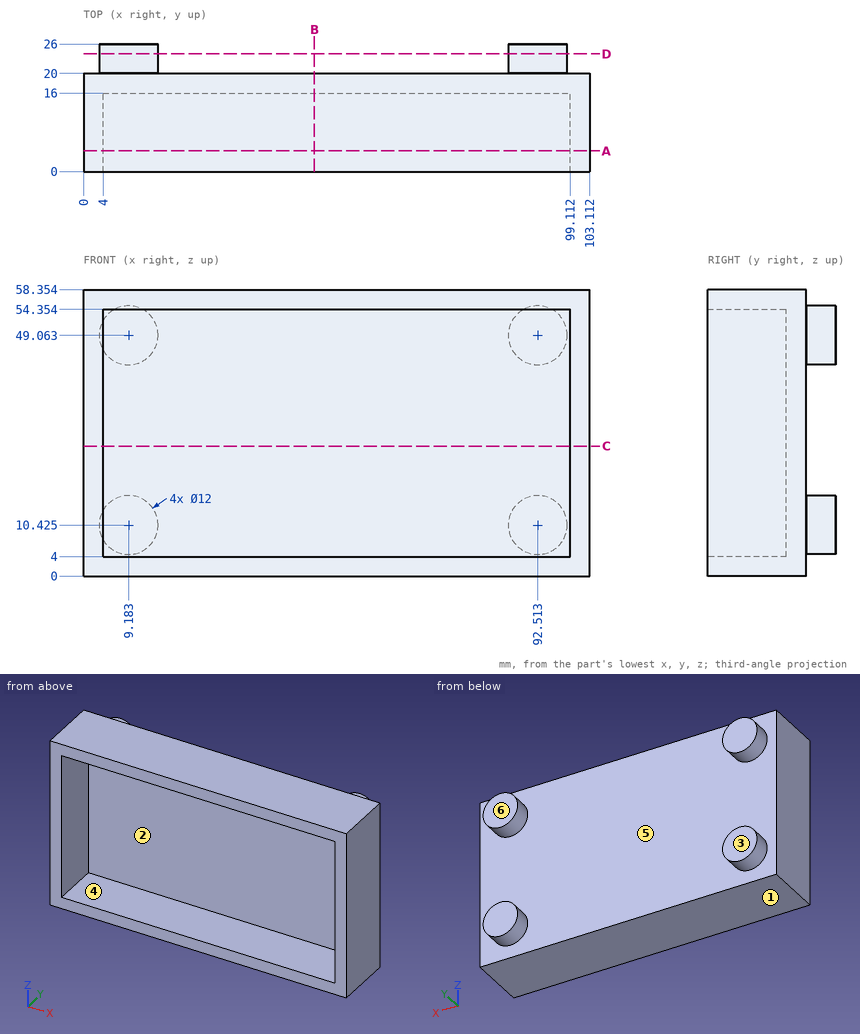
Could you check a few things on this drawing? It's one solid part, dimensions in mm from its lowest x, y, z. A direction names the side the tool comes from. Coordinates: 2 decimals unless noted, no trailing zeros. Loops run counter-clockwise (first coordinate to the right, second up) from the corner with the lowest first, then second, coordinate; pieces in that order, holes last. Notation, with made-up numbers: (42.5, 55.5) - (48.5, 55.5) arc R32 ccw to (48.5, 84.5) - close; hole circle Ø5 at (-10.5, 6). An arc over 180 degrees is marked (long way). Answer as a JSON object with one key per item and string values. Group by question number.
Item 1: On a 3-axis mill with a long thin cutter (end or side, diameter ignored), from which of +Z, -Z, +X, -X, +Y, -Y can I reach the whole of each face in a straight line? I mean the marked faces 4, 5 and 6. Say none if no direction works.
Item 2: If we section it at B-B (x = 47): List the corners of the cut face in (y, z) for me (1 decimal).
Item 3: If we section it at C-C (z = 26.5): List the corners of the cut face in (x, y) for me.
Item 4: If we section it at A-A (y = 4.25): List the corners of the cut face in (x, z) for me (1 decimal).
Item 5: If we mould it in two halves opening along Z, with no side actions, what happens to the marked faces 1, 2 and 3? For each: released by +Z, released by -Z, zero draft, split by the parting line, or undercut.
Item 6: For pin 1 (2 mm diameter, centred on x = 44, z = 9.5, fed in from -Y); pin 2 (17.5 mm diameter, centred on x = 46.5, z = 40.5, fed in from +Y); pin 3 (1 mm diameter, centred on y = 23, z = 11, fed in from +X); pin 4 (1.5 mm diameter, centred on x = 16.5, y = 21, fed in from +Z), each with a flat end and sliding along its axis, tell me the tip position at first contact or that it passes through.
Item 7: If we section it at D-D (y = 24): List the corners of the cut face in (x, z) for me (1 decimal).
Item 8: If I drill on L1, parallel to Z at x = 23, y = 12.5 (1 decimal); L2, parallel to X at y = 25, z = 49; L3, parallel to X at y = 14.25, z = 44.5, over which ranges is the centre line in solid material (lowest first)? Write a range as from..to.
Returned:
{
 "1": {"face 4": "-Y", "face 5": "+Y", "face 6": "+Z, -Z, +X, -X, +Y"},
 "2": {"outline": "(0, 0) - (20, 0) - (20, 58.4) - (0, 58.4) - (0, 54.4) - (16, 54.4) - (16, 4) - (0, 4) - close"},
 "3": {"outline": "(0, 0) - (4, 0) - (4, 16) - (99.11, 16) - (99.11, 0) - (103.11, 0) - (103.11, 20) - (0, 20) - close"},
 "4": {"outline": "(0, 0) - (103.1, 0) - (103.1, 58.4) - (0, 58.4) - close; hole (4, 4) - (99.1, 4) - (99.1, 54.4) - (4, 54.4) - close"},
 "5": {"face 1": "released by -Z", "face 2": "undercut", "face 3": "zero draft"},
 "6": {"pin 1": "stops at y = 16", "pin 2": "stops at y = 20", "pin 3": "stops at x = 98.51", "pin 4": "passes through"},
 "7": {"outline": "circle Ø12 at (9.2, 10.4); circle Ø12 at (9.2, 49.1); circle Ø12 at (92.5, 10.4); circle Ø12 at (92.5, 49.1)"},
 "8": {"L1": "z = 0..4, 54.4..58.4", "L2": "x = 3.18..15.18, 86.51..98.51", "L3": "x = 0..4, 99.11..103.11"}
}
